Autodesk Inventor part; units mm, degrees
ref_plane "YZ Plane" through (0, 0, 0) normal (1, 0, 0) x (0, 1, 0)
ref_plane "XZ Plane" through (0, 0, 0) normal (0, 1, 0) x (-1, 0, 0)
ref_plane "XY Plane" through (0, 0, 0) normal (0, 0, 1) x (1, 0, 0)
sketch "Sketch1" plane through (0, 0, 0) normal (0, 0, 1) x (1, 0, 0)
  line L0 (-164.322, 128.7031) -> (152.924, 128.7031)
  line L1 (152.924, 128.7031) -> (152.924, -133.4523)
  line L2 (152.924, -133.4523) -> (-164.322, -133.4523)
  line L3 (-164.322, -133.4523) -> (-164.322, 128.7031)
  point P0 (0, 0)
  dimension "d0" = 317.246
extrude "Extrusion1" add sketch "Sketch1" along normal blind 4.699
sketch "Sketch2" plane through (0, 0, 4.699) normal (0, 0, 1) x (1, 0, 0)
  line L0 (-22.7697, 25.1619) -> (2.6303, 25.1619)
  line L1 (52.3147, 22.4498) -> (52.3147, -24.5402)
  line L2 (-64.5253, -24.5402) -> (-64.5253, 22.4498)
  line L3 (52.3147, 22.4498) -> (54.8547, 22.4498)
  line L4 (54.8547, 22.4498) -> (54.8547, -24.5402)
  line L5 (54.8547, -24.5402) -> (52.3147, -24.5402)
  line L6 (52.3147, -24.5402) -> (52.3147, 22.4498)
  line L7 (-64.5253, -24.5402) -> (-67.0653, -24.5402)
  line L8 (-67.0653, -24.5402) -> (-67.0653, 22.4498)
  line L9 (-67.0653, 22.4498) -> (-64.5253, 22.4498)
  line L10 (-64.5253, 22.4498) -> (-64.5253, -24.5402)
  line L11 (-22.7697, 25.1619) -> (2.6303, 25.1619)
  line L12 (2.6303, 25.1619) -> (2.6303, 27.7019)
  line L13 (2.6303, 27.7019) -> (-22.7697, 27.7019)
  line L14 (-22.7697, 27.7019) -> (-22.7697, 25.1619)
  line L15 (-22.7697, -25.2309) -> (2.6303, -25.2309)
  line L16 (2.6303, -25.2309) -> (2.6303, -27.7709)
  line L17 (2.6303, -27.7709) -> (-22.7697, -27.7709)
  line L18 (-22.7697, -27.7709) -> (-22.7697, -25.2309)
  circle A0 centre (92.5652, 17.0242) radius 2.286
  circle A1 centre (100.1852, 17.0242) radius 2.286
  circle A2 centre (92.5652, -8.3758) radius 2.286
  circle A3 centre (100.1852, -8.3758) radius 2.286
  line L19 (3.9163, 100.2262) -> (59.1645, 100.2262)
  circle A4 centre (54.7163, 69.5732) radius 1.397
  circle A5 centre (54.7163, 117.8332) radius 1.397
  circle A6 centre (3.9163, 114.6403) radius 1.397
  circle A7 centre (3.9163, 86.7003) radius 1.397
  point P0 (0, 0)
  dimension "d3" = 116.84
  dimension "d4" = 46.99
  dimension "d5" = 2.54
  dimension "d6" = 2.54
  dimension "d7" = 25.4
  dimension "d8" = 2.54
  dimension "d9" = 2.54
  dimension "d12" = 4.572
  dimension "d31" = 25.4
  dimension "d32" = 25.4
extrude "Extrusion2" cut sketch "Sketch2" against normal blind 25.4
sketch "Sketch3" plane through (0, 0, 4.699) normal (0, 0, 1) x (1, 0, 0)
  line L0 (-164.322, 128.7031) -> (-164.322, -133.4523)
  line L1 (152.924, 128.7031) -> (152.924, -133.4523)
  line L2 (-164.322, -44.2248) -> (152.924, -44.2248)
  line L3 (152.924, -44.2248) -> (152.924, -133.4523)
  line L4 (152.924, -133.4523) -> (-164.322, -133.4523)
  line L5 (-164.322, -133.4523) -> (-164.322, -44.2248)
  point P0 (0, 0)
extrude "Extrusion3" cut sketch "Sketch3" against normal blind 25.4
sketch "Sketch4" plane through (0, 0, 4.699) normal (0, 0, 1) x (1, 0, 0)
  line L0 (-102.2349, 116.84) -> (-53.5128, 116.84)
  line L1 (-6.2523, 108.1454) -> (-6.2523, 44.8408)
  line L2 (-53.5128, 53.5354) -> (-102.2349, 53.5354)
  line L3 (-148.4923, 53.5354) -> (-148.4923, 108.1454)
  line L4 (-148.4923, 108.1454) -> (-151.0323, 108.1454)
  line L5 (-151.0323, 108.1454) -> (-151.0323, 53.5354)
  line L6 (-151.0323, 53.5354) -> (-148.4923, 53.5354)
  line L7 (-148.4923, 53.5354) -> (-148.4923, 108.1454)
  line L8 (-6.2523, 108.1454) -> (-3.7123, 108.1454)
  line L9 (-3.7123, 108.1454) -> (-3.7123, 53.5354)
  line L10 (-3.7123, 53.5354) -> (-6.2523, 53.5354)
  line L11 (-6.2523, 53.5354) -> (-6.2523, 108.1454)
  line L12 (-102.2349, 116.84) -> (-53.5128, 116.84)
  line L13 (-53.5128, 116.84) -> (-53.5128, 119.5161)
  line L14 (-53.5128, 119.5161) -> (-102.2349, 119.5161)
  line L15 (-102.2349, 119.5161) -> (-102.2349, 116.84)
  line L16 (-102.2349, 53.5354) -> (-53.5128, 53.5354)
  line L17 (-53.5128, 53.5354) -> (-53.5128, 50.5868)
  line L18 (-53.5128, 50.5868) -> (-102.2349, 50.5868)
  line L19 (-102.2349, 50.5868) -> (-102.2349, 53.5354)
  circle A0 centre (-100.2931, 0) radius 6.35
  point P0 (0, 0)
  dimension "d21" = 142.24
  dimension "d22" = 2.54
  dimension "d23" = 2.54
  dimension "d24" = 12.7
  dimension "d25" = 54.61
extrude "Extrusion4" cut sketch "Sketch4" against normal blind 25.4
sketch "Sketch5" plane through (0, 0, 4.699) normal (0, 0, 1) x (1, 0, 0)
  circle A0 centre (-154.2096, 125.6742) radius 4.064
  line L0 (-6.2523, 53.5354) -> (-6.2523, 108.1454)
  line L1 (-6.2523, 108.1454) -> (-3.7123, 108.1454)
  line L2 (-3.7123, 108.1454) -> (-3.7123, 53.5354)
  line L3 (-3.7123, 53.5354) -> (-6.2523, 53.5354)
  line L4 (-102.2349, 116.84) -> (-102.2349, 119.5161)
  line L5 (-102.2349, 119.5161) -> (-53.5128, 119.5161)
  line L6 (-53.5128, 119.5161) -> (-53.5128, 116.84)
  line L7 (-53.5128, 116.84) -> (-102.2349, 116.84)
  circle A1 centre (-100.2931, 0) radius 6.35
  line L8 (-151.0323, 53.5354) -> (-151.0323, 108.1454)
  line L9 (-151.0323, 108.1454) -> (-148.4923, 108.1454)
  line L10 (-148.4923, 108.1454) -> (-148.4923, 53.5354)
  line L11 (-148.4923, 53.5354) -> (-151.0323, 53.5354)
  line L12 (-102.2349, 53.5354) -> (-53.5128, 53.5354)
  line L13 (-53.5128, 53.5354) -> (-53.5128, 50.5868)
  line L14 (-53.5128, 50.5868) -> (-102.2349, 50.5868)
  line L15 (-102.2349, 50.5868) -> (-102.2349, 53.5354)
  line L16 (-164.322, -44.2248) -> (152.924, -44.2248)
  line L17 (152.924, -44.2248) -> (152.924, 128.7031)
  line L18 (152.924, 128.7031) -> (-164.322, 128.7031)
  line L19 (-164.322, 128.7031) -> (-164.322, -44.2248)
  line L20 (-164.322, 128.7031) -> (152.924, 128.7031)
  line L21 (-5.699, 128.7031) -> (-5.699, 116.84)
  circle A2 centre (145.9955, 120.8351) radius 4.064
  line L22 (-164.322, -44.2248) -> (-164.322, 128.7031)
  line L23 (-164.322, 42.2392) -> (-157.3936, 42.2392)
  circle A3 centre (-157.3936, -36.3568) radius 4.064
  circle A4 centre (145.9955, -36.3568) radius 4.064
  point P0 (0, 0)
  dimension "d28" = 8.128
extrude "Extrusion5" cut sketch "Sketch5" against normal blind 25.4 contours A0 L18 | L18 A0 | A2 | A3 | A4
sketch "Sketch6" plane through (0, 0, 4.699) normal (0, 0, 1) x (1, 0, 0)
  circle A0 centre (-157.3936, -36.3568) radius 4.064
  arc A1 (-156.9191, 128.7031) -> (-151.5, 128.7031) centre (-154.2096, 125.6742) ccw
  circle A2 centre (145.9955, 120.8351) radius 4.064
  circle A3 centre (145.9955, -36.3568) radius 4.064
  line L0 (-6.2523, 53.5354) -> (-6.2523, 108.1454)
  line L1 (-6.2523, 108.1454) -> (-3.7123, 108.1454)
  line L2 (-3.7123, 108.1454) -> (-3.7123, 53.5354)
  line L3 (-3.7123, 53.5354) -> (-6.2523, 53.5354)
  line L4 (-102.2349, 116.84) -> (-102.2349, 119.5161)
  line L5 (-102.2349, 119.5161) -> (-53.5128, 119.5161)
  line L6 (-53.5128, 119.5161) -> (-53.5128, 116.84)
  line L7 (-53.5128, 116.84) -> (-102.2349, 116.84)
  circle A4 centre (-100.2931, 0) radius 6.35
  line L8 (-151.0323, 53.5354) -> (-151.0323, 108.1454)
  line L9 (-151.0323, 108.1454) -> (-148.4923, 108.1454)
  line L10 (-148.4923, 108.1454) -> (-148.4923, 53.5354)
  line L11 (-148.4923, 53.5354) -> (-151.0323, 53.5354)
  line L12 (-102.2349, 53.5354) -> (-53.5128, 53.5354)
  line L13 (-53.5128, 53.5354) -> (-53.5128, 50.5868)
  line L14 (-53.5128, 50.5868) -> (-102.2349, 50.5868)
  line L15 (-102.2349, 50.5868) -> (-102.2349, 53.5354)
  line L16 (-164.322, -44.2248) -> (152.924, -44.2248)
  line L17 (152.924, -44.2248) -> (152.924, 128.7031)
  line L18 (152.924, 128.7031) -> (-151.5, 128.7031)
  line L19 (-164.322, 128.7031) -> (-164.322, -44.2248)
  line L20 (-64.5253, 22.4498) -> (-64.5253, -24.5402)
  line L21 (-64.5253, -24.5402) -> (-67.0653, -24.5402)
  line L22 (-67.0653, -24.5402) -> (-67.0653, 22.4498)
  line L23 (-67.0653, 22.4498) -> (-64.5253, 22.4498)
  line L24 (-22.7697, -27.7709) -> (-22.7697, -25.2309)
  line L25 (-22.7697, -25.2309) -> (2.6303, -25.2309)
  line L26 (2.6303, -25.2309) -> (2.6303, -27.7709)
  line L27 (2.6303, -27.7709) -> (-22.7697, -27.7709)
  circle A5 centre (100.1852, -8.3758) radius 2.286
  circle A6 centre (100.1852, 17.0242) radius 2.286
  circle A7 centre (54.7163, 117.8332) radius 1.397
  circle A8 centre (54.7163, 69.5732) radius 1.397
  circle A9 centre (3.9163, 86.7003) radius 1.397
  circle A10 centre (3.9163, 114.6403) radius 1.397
  circle A11 centre (92.5652, 17.0242) radius 2.286
  circle A12 centre (92.5652, -8.3758) radius 2.286
  line L28 (-22.7697, 25.1619) -> (-22.7697, 27.7019)
  line L29 (-22.7697, 27.7019) -> (2.6303, 27.7019)
  line L30 (2.6303, 27.7019) -> (2.6303, 25.1619)
  line L31 (2.6303, 25.1619) -> (-22.7697, 25.1619)
  line L32 (52.3147, -24.5402) -> (52.3147, 22.4498)
  line L33 (52.3147, 22.4498) -> (54.8547, 22.4498)
  line L34 (54.8547, 22.4498) -> (54.8547, -24.5402)
  line L35 (54.8547, -24.5402) -> (52.3147, -24.5402)
  line L36 (-164.322, 128.7031) -> (152.924, 128.7031)
  line L37 (-164.322, 128.7031) -> (152.924, 128.7031)
  line L38 (152.924, 128.7031) -> (152.924, 136.3029)
  line L39 (152.924, 136.3029) -> (-164.322, 136.3029)
  line L40 (-164.322, 136.3029) -> (-164.322, 128.7031)
  line L41 (-156.9191, 128.7031) -> (-164.322, 128.7031)
  point P0 (0, 0)
extrude "Extrusion6" add sketch "Sketch6" against normal blind 4.699 contours L36 L40 L39 L38 L18
sketch "Sketch7" plane through (0, 0, 4.699) normal (0, 0, 1) x (1, 0, 0)
  arc A0 (-156.9191, 128.7031) -> (-151.5, 128.7031) centre (-154.2096, 125.6742) ccw
  line L0 (-156.9191, 128.7031) -> (-151.5, 128.7031)
  line L1 (152.924, -44.2248) -> (152.924, 136.3029)
  line L2 (152.924, 136.3029) -> (-164.322, 136.3029)
  line L3 (-164.322, 136.3029) -> (-164.322, -44.2248)
  line L4 (-164.322, -44.2248) -> (152.924, -44.2248)
  circle A1 centre (-157.3936, -36.3568) radius 4.064
  circle A2 centre (145.9955, 120.8351) radius 4.064
  circle A3 centre (145.9955, -36.3568) radius 4.064
  line L5 (-6.2523, 53.5354) -> (-6.2523, 108.1454)
  line L6 (-6.2523, 108.1454) -> (-3.7123, 108.1454)
  line L7 (-3.7123, 108.1454) -> (-3.7123, 53.5354)
  line L8 (-3.7123, 53.5354) -> (-6.2523, 53.5354)
  line L9 (-102.2349, 116.84) -> (-102.2349, 119.5161)
  line L10 (-102.2349, 119.5161) -> (-53.5128, 119.5161)
  line L11 (-53.5128, 119.5161) -> (-53.5128, 116.84)
  line L12 (-53.5128, 116.84) -> (-102.2349, 116.84)
  circle A4 centre (-100.2931, 0) radius 6.35
  line L13 (-151.0323, 53.5354) -> (-151.0323, 108.1454)
  line L14 (-151.0323, 108.1454) -> (-148.4923, 108.1454)
  line L15 (-148.4923, 108.1454) -> (-148.4923, 53.5354)
  line L16 (-148.4923, 53.5354) -> (-151.0323, 53.5354)
  line L17 (-102.2349, 53.5354) -> (-53.5128, 53.5354)
  line L18 (-53.5128, 53.5354) -> (-53.5128, 50.5868)
  line L19 (-53.5128, 50.5868) -> (-102.2349, 50.5868)
  line L20 (-102.2349, 50.5868) -> (-102.2349, 53.5354)
  line L21 (-64.5253, 22.4498) -> (-64.5253, -24.5402)
  line L22 (-64.5253, -24.5402) -> (-67.0653, -24.5402)
  line L23 (-67.0653, -24.5402) -> (-67.0653, 22.4498)
  line L24 (-67.0653, 22.4498) -> (-64.5253, 22.4498)
  line L25 (-22.7697, -27.7709) -> (-22.7697, -25.2309)
  line L26 (-22.7697, -25.2309) -> (2.6303, -25.2309)
  line L27 (2.6303, -25.2309) -> (2.6303, -27.7709)
  line L28 (2.6303, -27.7709) -> (-22.7697, -27.7709)
  circle A5 centre (100.1852, -8.3758) radius 2.286
  circle A6 centre (100.1852, 17.0242) radius 2.286
  circle A7 centre (54.7163, 117.8332) radius 1.397
  circle A8 centre (54.7163, 69.5732) radius 1.397
  circle A9 centre (3.9163, 86.7003) radius 1.397
  circle A10 centre (3.9163, 114.6403) radius 1.397
  circle A11 centre (92.5652, 17.0242) radius 2.286
  circle A12 centre (92.5652, -8.3758) radius 2.286
  line L29 (-22.7697, 25.1619) -> (-22.7697, 27.7019)
  line L30 (-22.7697, 27.7019) -> (2.6303, 27.7019)
  line L31 (2.6303, 27.7019) -> (2.6303, 25.1619)
  line L32 (2.6303, 25.1619) -> (-22.7697, 25.1619)
  line L33 (52.3147, -24.5402) -> (52.3147, 22.4498)
  line L34 (52.3147, 22.4498) -> (54.8547, 22.4498)
  line L35 (54.8547, 22.4498) -> (54.8547, -24.5402)
  line L36 (54.8547, -24.5402) -> (52.3147, -24.5402)
  circle A13 centre (-154.2096, 125.6742) radius 4.064
  point P0 (0, 0)
properties part number "bottom"
Could you check a few things on this model? Use its own coordinates, in mm. Give positions to 0.01 mm unless a question says otherwise; leave off trailing zeros. Order: outer loops, then holes, each group sorted by start corner. A loop starts at its lowest first (then second) coordinate and runs counter-clockwise, first axis right, second up.
1. Suppose I cut it at C-C (x = -9.5). List the corners of the cut face in (y, z) for me.
2. Suppose I cut it at A-A (y = 0). List the corners of the cut face in (x, z) for me, plus the area to 3 significant figures.
3. Suppose I cut it at B-B (x = -83). List the corners of the cut face in (y, z) for me, plus the area to 3 significant figures.
4. Suppose I cut it at D-D (z = 3.5). Give the number of separate pieces and of enclosed holes in the cut face, plus the area to 3 significant figures.
5. I need wall thicknesses on L1, parallel to X at y = 98, z = 3.7; L2, parallel to Y at x = -101, z = 0.7; L3, parallel to Y at x = 100.5, z = 3.6. Which ranges of each line are inside material? Lowest first, please.
6. We'd pull the mould along X, two halves only. Please class faces 1 (the cylindrical face through (-104.973, 4.292, 2.382)), 2 (the flat face through (-8, 47, 4.699)): pulls with the +X half, pulls with the -X half, needs draft (parallel to the pull), parting line crosses it, or undercut.
Solved:
1. outline: (-44.22, 0) - (-27.77, 0) - (-27.77, 4.7) - (-44.22, 4.7) - close; (-25.23, 0) - (25.16, 0) - (25.16, 4.7) - (-25.23, 4.7) - close; (27.7, 0) - (136.3, 0) - (136.3, 4.7) - (27.7, 4.7) - close
2. outline: (-164.32, 0) - (-106.64, 0) - (-106.64, 4.7) - (-164.32, 4.7) - close; (-93.94, 0) - (-67.07, 0) - (-67.07, 4.7) - (-93.94, 4.7) - close; (-64.53, 0) - (52.31, 0) - (52.31, 4.7) - (-64.53, 4.7) - close; (54.85, 0) - (152.92, 0) - (152.92, 4.7) - (54.85, 4.7) - close
2. area: 1,410 mm2
3. outline: (-44.22, 0) - (50.59, 0) - (50.59, 4.7) - (-44.22, 4.7) - close; (53.54, 0) - (116.84, 0) - (116.84, 4.7) - (53.54, 4.7) - close; (119.52, 0) - (136.3, 0) - (136.3, 4.7) - (119.52, 4.7) - close
3. area: 822 mm2
4. separate pieces: 1
4. enclosed holes: 21
4. area: 55,900 mm2
5. L1: x = -164.32 to -151.03, -148.49 to -6.25, -3.71 to 152.92
5. L2: y = -44.22 to -6.31, 6.31 to 50.59, 53.54 to 116.84, 119.52 to 136.3
5. L3: y = -44.22 to -10.64, -6.11 to 14.76, 19.29 to 136.3
6. face 1: undercut
6. face 2: needs draft
